```python
from build123d import *

# Parameters (mm, degrees)
F0_W     = 250
F0_H     = 9
F0_R     = 1.075
F1_DEPTH = 8
F2_W     = 4.2
F2_H     = 5.3
F3_DEPTH = 12
F4_W     = 2.1
F4_H     = 4
F5_DEPTH = 4.5


with BuildPart() as f1:
    # F0 (on Front) → F1 (new body)
    with BuildSketch(Plane.XZ):
        with Locations((125, 4.5)):
            Rectangle(F0_W, F0_H)
        with Locations((10, 4.5)):
            Circle(F0_R, mode=Mode.SUBTRACT)
        with Locations((20, 4.5)):
            Circle(F0_R, mode=Mode.SUBTRACT)
        with Locations((30, 4.5)):
            Circle(F0_R, mode=Mode.SUBTRACT)
        with Locations((40, 4.5)):
            Circle(F0_R, mode=Mode.SUBTRACT)
        with Locations((50, 4.5)):
            Circle(F0_R, mode=Mode.SUBTRACT)
        with Locations((60, 4.5)):
            Circle(F0_R, mode=Mode.SUBTRACT)
        with Locations((70, 4.5)):
            Circle(F0_R, mode=Mode.SUBTRACT)
        with Locations((80, 4.5)):
            Circle(F0_R, mode=Mode.SUBTRACT)
        with Locations((90, 4.5)):
            Circle(F0_R, mode=Mode.SUBTRACT)
        with Locations((100, 4.5)):
            Circle(F0_R, mode=Mode.SUBTRACT)
        with Locations((110, 4.5)):
            Circle(F0_R, mode=Mode.SUBTRACT)
        with Locations((120, 4.5)):
            Circle(F0_R, mode=Mode.SUBTRACT)
        with Locations((130, 4.5)):
            Circle(F0_R, mode=Mode.SUBTRACT)
        with Locations((140, 4.5)):
            Circle(F0_R, mode=Mode.SUBTRACT)
        with Locations((150, 4.5)):
            Circle(F0_R, mode=Mode.SUBTRACT)
        with Locations((160, 4.5)):
            Circle(F0_R, mode=Mode.SUBTRACT)
        with Locations((170, 4.5)):
            Circle(F0_R, mode=Mode.SUBTRACT)
        with Locations((180, 4.5)):
            Circle(F0_R, mode=Mode.SUBTRACT)
        with Locations((190, 4.5)):
            Circle(F0_R, mode=Mode.SUBTRACT)
        with Locations((200, 4.5)):
            Circle(F0_R, mode=Mode.SUBTRACT)
        with Locations((210, 4.5)):
            Circle(F0_R, mode=Mode.SUBTRACT)
        with Locations((220, 4.5)):
            Circle(F0_R, mode=Mode.SUBTRACT)
        with Locations((230, 4.5)):
            Circle(F0_R, mode=Mode.SUBTRACT)
        with Locations((240, 4.5)):
            Circle(F0_R, mode=Mode.SUBTRACT)
    extrude(amount=F1_DEPTH)

    # F2 (on face) → F3 (cut)
    with BuildSketch(Plane.YZ.offset(250)):
        with Locations((-4, 4.5)):
            Rectangle(F2_W, F2_H)
    extrude(amount=-F3_DEPTH, mode=Mode.SUBTRACT)

    # F4 (on face) → F5 (cut)
    with BuildSketch(Plane(origin=(0, 0, 0), x_dir=(-1, 0, 0), z_dir=(0, 1, 0))):
        with Locations((-15.05, 4.5)):
            Rectangle(F4_W, F4_H)
        with Locations((-45.05, 4.5)):
            Rectangle(F4_W, F4_H)
        with Locations((-75.05, 4.5)):
            Rectangle(F4_W, F4_H)
        with Locations((-105.05, 4.5)):
            Rectangle(F4_W, F4_H)
        with Locations((-135.05, 4.5)):
            Rectangle(F4_W, F4_H)
        with Locations((-165.05, 4.5)):
            Rectangle(F4_W, F4_H)
        with Locations((-195.05, 4.5)):
            Rectangle(F4_W, F4_H)
        with Locations((-225.05, 4.5)):
            Rectangle(F4_W, F4_H)
    extrude(amount=-F5_DEPTH, mode=Mode.SUBTRACT)


solid = f1.part
```
For this review, take the finished solid that the model builds, in its own axes (mm). A direction names the side the tool comes from. Round coordinates to 2 decimals unless told otherwise and drop trailing zeros. Write each question's results on one line, items separated by ' | '.
Item 1: For pin 1 (1.9 mm diameter, centred on x = 40, z = 4.5, fed in from +Y); pin 2 (2 mm diameter, centred on y = -3, z = 5.5, fed in from +X); pin 3 (0.6 mm diameter, centred on x = 45.5, z = 4.5, fed in from +Y), all flat-tipped, find the tip position at first contact; note any pin that passes through.
Calculated:
pin 1: passes through | pin 2: stops at x = 238 | pin 3: stops at y = -4.5
Item 2: To check wall thickness, follow line 1 along Z through (x, y) = (30, -4) (3 decimals); line 2 along Z through (x, y) = (105.5, -0.75); line 3 along X through (y, z) = (-2.5, 2.25). State the ranges of each line that lie inside material, in increasing order. Write a range as from..to.
Calculated:
line 1: z = 0..3.425, 5.575..9 | line 2: z = 0..2.5, 6.5..9 | line 3: x = 0..238
Item 3: Draft analysis for pull direction X (two halves, no side actions). For faces 1 (the face through (123, -4, 9)), 2 (the face through (250, -7, 4)), 3 (the face through (194, -2, 4)), state which applies: pulls with the +X half, pulls with the -X half, needs draft (parallel to the pull), parting line crosses it, or undercut.
Calculated:
face 1: needs draft | face 2: pulls with the +X half | face 3: undercut
Item 4: For faces 4 (the face through (74, -2, 4)), 5 (the face through (244, -4, 7.15)), 6 (the face through (123, -4, 0)), list the 3-axis set-ups (+Z, -Z, +X, -X, +Y, -Y) from which the entire face can be reached by the end or side of a thin tool; tool diameter is ignored.
Calculated:
face 4: +Y | face 5: +X | face 6: -Z, +X, -X, +Y, -Y
